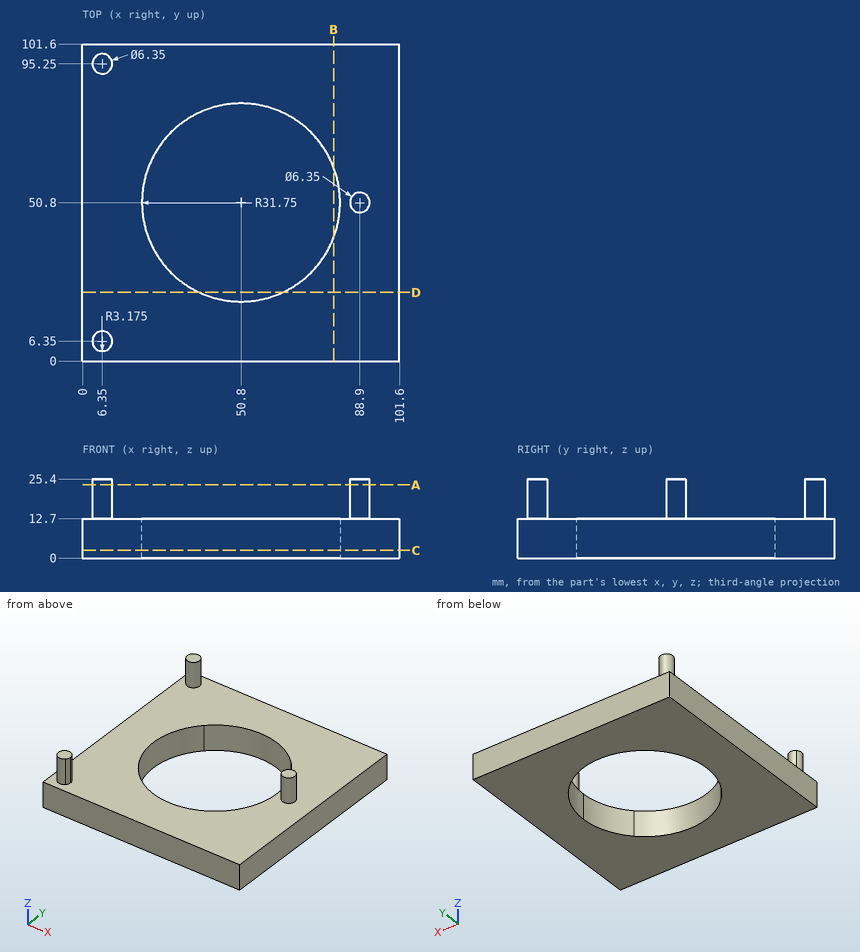
Geometry: see drawing. Coordinates: mm, zero at the bounding-box minimum. Give positions to 0.01 mm unless a question says otherwise; leave off trailing zeros. Order: outer loops, then holes, each group sorted by start corner. A loop starts at its lowest first (then second) coordinate and runs counter-clockwise, first axis right, second up. Notation, with made-up numbers: (-25.5, 79) - (10.5, 79) arc R14 ccw to (10.5, 97) - close; hole circle Ø5 at (36.5, 40). An arc over 180 degrees is marked (long way). One line per item, written item: value.
1. Cut plane C-C, the plane z = 2.5. Output: boundary loops of the cut face in (x, y), and give its area (3 significant figures).
Determined:
outline: (0, 0) - (101.6, 0) - (101.6, 101.6) - (0, 101.6) - close; hole circle Ø63.5 at (50.8, 50.8)
area: 7,160 mm2
2. Cut plane B-B, the plane x = 80.5. Output: boundary loops of the cut face in (y, z).
Determined:
outline: (0, 0) - (39.58, 0) - (39.58, 12.7) - (0, 12.7) - close; (62.02, 0) - (101.6, 0) - (101.6, 12.7) - (62.02, 12.7) - close
3. Cut plane D-D, the plane y = 22. Output: boundary loops of the cut face in (x, z), and give its area (3 significant figures).
Determined:
outline: (0, 0) - (37.44, 0) - (37.44, 12.7) - (0, 12.7) - close; (64.16, 0) - (101.6, 0) - (101.6, 12.7) - (64.16, 12.7) - close
area: 951 mm2
4. Cut plane A-A, the plane z = 23.5. Output: boundary loops of the cut face in (x, y) (3 decimals), and give its area (3 significant figures).
Determined:
outline: circle Ø6.35 at (6.35, 6.35); circle Ø6.35 at (6.35, 95.25); circle Ø6.35 at (88.9, 50.8)
area: 95.0 mm2
5. Line query: probe 1 along Z at (x, y) = (29, 27); probe 2 along Y at (x, z) = (31.5, 11.75); probe 3 along X at (y, z) = (51.5, 9). Output: solid intervals per line, ascending.
Determined:
probe 1: 0 to 12.7
probe 2: 0 to 25.59, 76.01 to 101.6
probe 3: 0 to 19.06, 82.54 to 101.6
6. Pin query (flat end, axial travel): pin 1 Ø4 at (x, z) = (50, 12.5) entering from -Y; pin 2 Ø12 at (y, z) = (58, 22.5) entering from -X; pin 3 Ø5 at (y, z) = (81, 17) entering from +X. Return the tip coordinate at first contact, or that it passes through.
Determined:
pin 1: y = 0
pin 2: x = 85.96
pin 3: through
